Print and shaded views of the part. All mm, measured from the part's lowest x, y and z. Round coordinates to 2 decimals unless told otherwise and drop trailing zeros. Order: outer loops, then holes, each group sorted by start corner. A loop starts at its lowest first (then second) coordinate and runs counter-clockwise, first axis right, second up. Notation, with made-up numbers: (74, 53.5) - (106, 53.5) arc R8 ccw to (106, 67.5) - close; hole circle Ø8 at (-36.5, -13.75). An arc over 180 degrees is marked (long way). Return JSON: item names as keys, results as strings. Group by question number.
Item 1: Two-plate mould, pull along Z, no slides. Class the marked faces 1, 2 and 3: released by +Z, released by -Z, zero draft, split by the parting line, or undercut.
Item 2: Saw through at D-D on x = 7. List the corners of the cut face in (y, z).
Item 3: Saw through at B-B on y = 18.5. List the corners of the cut face in (x, z) (1 decimal).
Item 4: Saw through at A-A on z = 34.5. List the corners of the cut face in (x, y), and give its area (3 significant figures).
Item 5: Probe probe 1 along Z at (x, y) = (29.5, 17.75) (1 decimal); probe 2 along Z at (x, y) = (37, 8) (1 decimal); probe 3 along X at (y, z) = (10.5, 34.5). List the from-to ranges inside material, lowest first.
Item 6: Drop flat-ended pins along their axis: pin 1 (12 mm diameter, centred on y = 4.5, z = 42, fed in from -X); pin 2 (3 mm diameter, centred on x = 49.5, y = 6, fed in from -Z) (1 decimal); pin 3 (6 mm diameter, centred on x = 11.5, y = 13, fed in from -Z) (1 decimal). Give the stop position or say it passes through.
Item 7: Saw through at C-C on z = 13.5. List the corners of the cut face in (x, y).
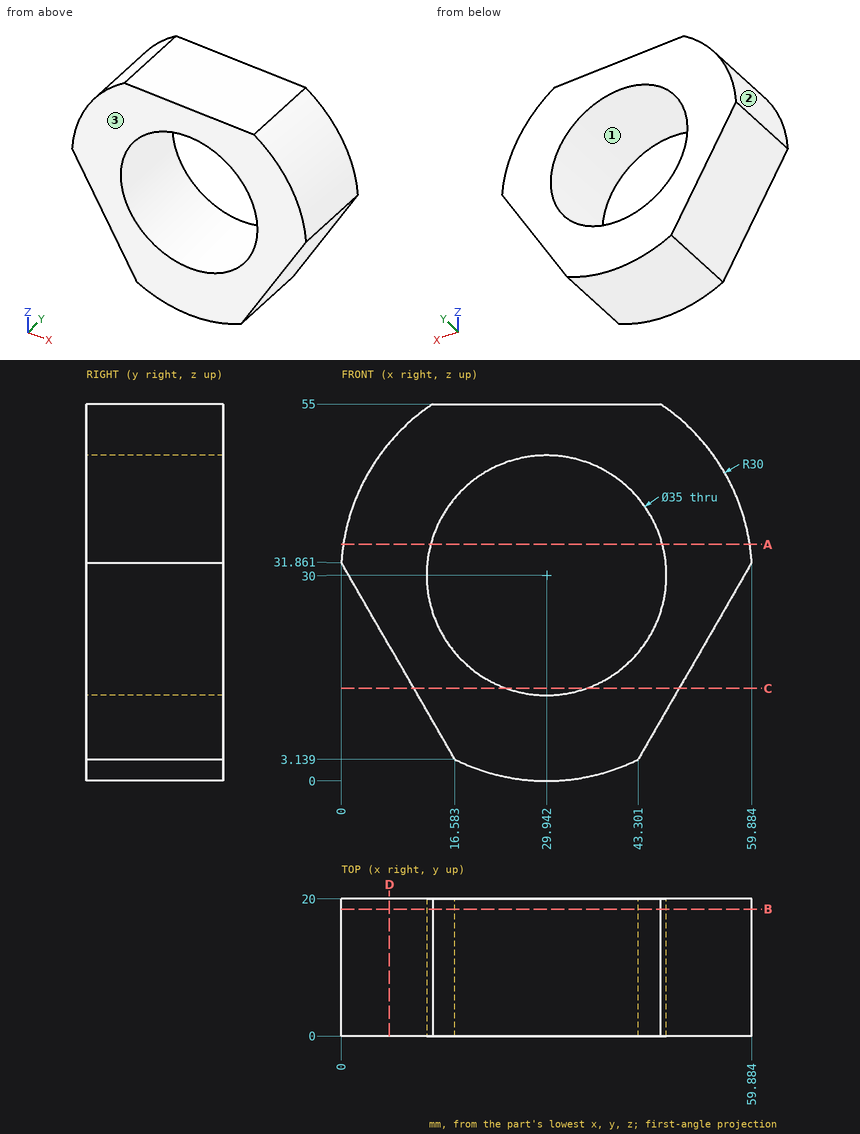
Filled in:
{
 "1": {"face 1": "undercut", "face 2": "released by +Z", "face 3": "zero draft"},
 "2": {"outline": "(0, 19.74) - (20, 19.74) - (20, 49.33) - (0, 49.33) - close"},
 "3": {"outline": "(0, 31.9) - (16.6, 3.1) arc R30 ccw to (43.3, 3.1) - (59.9, 31.9) arc R30 ccw to (46.5, 55) - (13.4, 55) arc R30 ccw to start; hole circle Ø35 at (29.9, 30)"},
 "4": {"outline": "(0.28, 0) - (13.03, 0) - (13.03, 20) - (0.28, 20) - close; (46.85, 0) - (59.6, 0) - (59.6, 20) - (46.85, 20) - close", "area": "510 mm^2"},
 "5": {"probe 1": "z = 0 to 12.5, 47.5 to 55", "probe 2": "z = 0.8 to 14, 46 to 55", "probe 3": "x = 0.28 to 13.03, 46.85 to 59.6"},
 "6": {"pin 1": "stops at x = 0.55", "pin 2": "stops at z = 11.3", "pin 3": "stops at z = 6.7"},
 "7": {"outline": "(10.6, 0) - (24.11, 0) - (24.11, 20) - (10.6, 20) - close; (35.77, 0) - (49.28, 0) - (49.28, 20) - (35.77, 20) - close"}
}
